from build123d import *

# Parameters (mm, degrees)
F1_DEPTH = 1.5748
F2_R     = 0.381
F3_DEPTH = 1.5758


with BuildPart() as f1:
    # F0 (on Top) → F1 (new body)
    with BuildSketch(Plane.XY):
        Polygon((0, 6.096), (0, 0), (25.3238, 0), (25.3238, 6.477), (26.0858, 6.477), (26.0858, 0), (97.536, 0), (97.536, 24.13), (26.0858, 24.13), (26.0858, 17.653), (25.3238, 17.653), (25.3238, 24.13), (0, 24.13), (0, 18.034), (-11.43, 18.034), (-11.43, 6.096), align=None)
    extrude(amount=F1_DEPTH)

    # F2 (on face) → F3 (cut, through all)
    with BuildSketch(Plane.XY.offset(1.5748)):
        with Locations((31.496, 1.905)):
            Circle(F2_R)
        with Locations((31.496, 22.225)):
            Circle(F2_R)
        with Locations((34.036, 1.905)):
            Circle(F2_R)
        with Locations((34.036, 22.225)):
            Circle(F2_R)
        with Locations((36.576, 1.905)):
            Circle(F2_R)
        with Locations((36.576, 22.225)):
            Circle(F2_R)
        with Locations((39.116, 1.905)):
            Circle(F2_R)
        with Locations((39.116, 22.225)):
            Circle(F2_R)
        with Locations((41.656, 1.905)):
            Circle(F2_R)
        with Locations((41.656, 22.225)):
            Circle(F2_R)
        with Locations((44.196, 1.905)):
            Circle(F2_R)
        with Locations((44.196, 22.225)):
            Circle(F2_R)
        with Locations((46.736, 1.905)):
            Circle(F2_R)
        with Locations((46.736, 22.225)):
            Circle(F2_R)
        with Locations((49.276, 1.905)):
            Circle(F2_R)
        with Locations((49.276, 22.225)):
            Circle(F2_R)
        with Locations((51.816, 1.905)):
            Circle(F2_R)
        with Locations((51.816, 22.225)):
            Circle(F2_R)
        with Locations((54.356, 1.905)):
            Circle(F2_R)
        with Locations((54.356, 22.225)):
            Circle(F2_R)
        with Locations((56.896, 1.905)):
            Circle(F2_R)
        with Locations((56.896, 22.225)):
            Circle(F2_R)
        with Locations((59.436, 1.905)):
            Circle(F2_R)
        with Locations((59.436, 22.225)):
            Circle(F2_R)
        with Locations((61.976, 1.905)):
            Circle(F2_R)
        with Locations((61.976, 22.225)):
            Circle(F2_R)
        with Locations((64.516, 1.905)):
            Circle(F2_R)
        with Locations((64.516, 22.225)):
            Circle(F2_R)
        with Locations((67.056, 1.905)):
            Circle(F2_R)
        with Locations((67.056, 22.225)):
            Circle(F2_R)
        with Locations((69.596, 1.905)):
            Circle(F2_R)
        with Locations((69.596, 22.225)):
            Circle(F2_R)
        with Locations((72.136, 1.905)):
            Circle(F2_R)
        with Locations((72.136, 22.225)):
            Circle(F2_R)
        with Locations((74.676, 1.905)):
            Circle(F2_R)
        with Locations((74.676, 22.225)):
            Circle(F2_R)
        with Locations((77.216, 1.905)):
            Circle(F2_R)
        with Locations((77.216, 22.225)):
            Circle(F2_R)
        with Locations((79.756, 1.905)):
            Circle(F2_R)
        with Locations((79.756, 22.225)):
            Circle(F2_R)
        with Locations((82.296, 1.905)):
            Circle(F2_R)
        with Locations((82.296, 22.225)):
            Circle(F2_R)
        with Locations((84.836, 1.905)):
            Circle(F2_R)
        with Locations((84.836, 22.225)):
            Circle(F2_R)
        with Locations((87.376, 1.905)):
            Circle(F2_R)
        with Locations((87.376, 22.225)):
            Circle(F2_R)
        with Locations((89.916, 1.905)):
            Circle(F2_R)
        with Locations((89.916, 22.225)):
            Circle(F2_R)
        with Locations((92.456, 1.905)):
            Circle(F2_R)
        with Locations((92.456, 22.225)):
            Circle(F2_R)
        with Locations((94.996, 1.905)):
            Circle(F2_R)
        with Locations((94.996, 22.225)):
            Circle(F2_R)
    extrude(amount=-F3_DEPTH, mode=Mode.SUBTRACT)


solid = f1.part
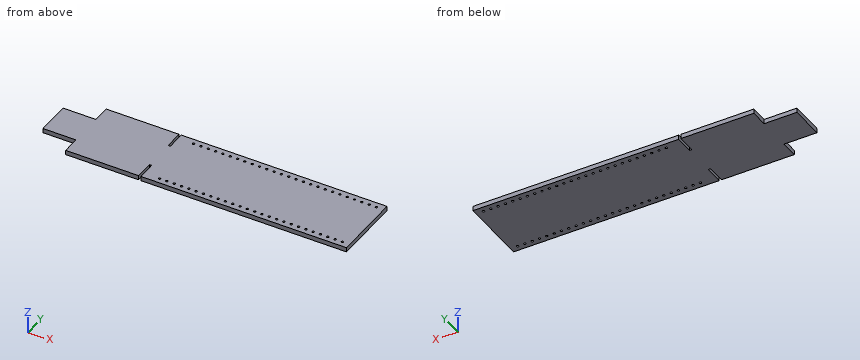
Geometry: final body of the model. Coordinates: model frame, mm. Give positions to 0.01 mm unless a question says otherwise; leave off trailing zeros. Loops run counter-clockwise (first coordinate to the right, second up) from the corner with the lowest first, then second, coordinate; pieces in that order, holes last. Notation, with made-up numbers: M 82,-11 L 86,-11 A13 cw 86,9 Z; hole C 82,64.5 d8. An arc over 180 degrees is marked long. Put each result on its own line as item: value.
1) Material intervals for L1, parallel to Y at x = 90, z = 1.3; L2, parallel to Y at x = 62, z = 0.3; L3, parallel to X at y = 6, z = 1, sorted ascending. Write a range as from..to.
Computed values:
L1: y = 0..1.53, 2.28..21.85, 22.6..24.13
L2: y = 0..1.52, 2.29..21.84, 22.61..24.13
L3: x = 0..25.32, 26.09..97.54
2) Cut plane A-A, the plane y = 19.5. Return the cut outline in (x, z), plus the area to 3 significant figures.
Computed values:
outline: M 0,0 L 25.32,0 L 25.32,1.57 L 0,1.57 Z; M 26.09,0 L 97.54,0 L 97.54,1.57 L 26.09,1.57 Z
area: 152 mm^2
3) First-contact query: P1, Ø0.5, axis at y = 21.5, z = 1, coming from the -X side. Flat tip, straight axial feed; report the tip coordinate or a pass-through.
Computed values:
P1: stops at x = 0
4) Cut plane B-B, the plane z = 1.1. Give the number of separate pieces and of enclosed holes in the cut face, plus the area to 3 significant figures.
Computed values:
separate pieces: 1
enclosed holes: 52
area: 2,460 mm^2
